from build123d import *

# Parameters (mm, degrees)
SKETCH1_W            = 21.082
SKETCH1_H            = 10.16
BOSS_EXTRUDE1_DEPTH  = 1.651
CUT_EXTRUDE1_DEPTH   = 22.082
MIRROR2_COPY_1_DEPTH = 22.082
CUT_EXTRUDE2_DEPTH   = 11.16
MIRROR4_COPY_1_DEPTH = 11.16
SKETCH4_R            = 0.5
CUT_EXTRUDE3_DEPTH   = 0.1


with BuildPart() as part:
    # Sketch1 → Boss-Extrude1 (new body, symmetric)
    with BuildSketch(Plane(origin=(0, 0, 0), x_dir=(1, 0, 0), z_dir=(0, 1, 0))):
        Rectangle(SKETCH1_W, SKETCH1_H)
    extrude(amount=BOSS_EXTRUDE1_DEPTH, both=True)

    # Sketch2 → Cut-Extrude1 (cut, through all)
    with BuildSketch(Plane(origin=(10.541, 0, 0), x_dir=(0, 0, -1), z_dir=(1, 0, 0))):
        Polygon((-5.08, 1.651), (-4.88, 1.651), (-5.08, 0.1905), align=None)
    cut_extrude1 = extrude(amount=-CUT_EXTRUDE1_DEPTH, mode=Mode.SUBTRACT)

    # Mirror1: Cut-Extrude1 across plane
    add(cut_extrude1.mirror(Plane.XY), mode=Mode.SUBTRACT)

    # Mirror2: Cut-Extrude1 across plane
    add(cut_extrude1.mirror(Plane.ZX), mode=Mode.SUBTRACT)

    # Mirror2 copy 1 sketch → Mirror2 copy 1 (cut, through all)
    with BuildSketch(Plane(origin=(10.541, 0, 0), x_dir=(0, 0, 1), z_dir=(1, 0, 0))):
        Polygon((-5.08, 1.651), (-4.88, 1.651), (-5.08, 0.1905), align=None)
    extrude(amount=-MIRROR2_COPY_1_DEPTH, mode=Mode.SUBTRACT)

    # Sketch3 → Cut-Extrude2 (cut, through all)
    with BuildSketch(Plane.XY.offset(5.08)):
        Polygon((10.541, 0.1905), (10.541, 1.651), (10.341, 1.651), align=None)
    cut_extrude2 = extrude(amount=-CUT_EXTRUDE2_DEPTH, mode=Mode.SUBTRACT)

    # Mirror3: Cut-Extrude2 across plane
    add(cut_extrude2.mirror(Plane.ZX), mode=Mode.SUBTRACT)

    # Mirror4: Cut-Extrude2 across plane
    add(cut_extrude2.mirror(Plane(origin=(0, 0, 0), x_dir=(0, 0, 1), z_dir=(1, 0, 0))), mode=Mode.SUBTRACT)

    # Mirror4 copy 1 sketch → Mirror4 copy 1 (cut, through all)
    with BuildSketch(Plane(origin=(0, 0, 5.08), x_dir=(-1, 0, 0), z_dir=(0, 0, 1))):
        Polygon((10.541, 0.1905), (10.541, 1.651), (10.341, 1.651), align=None)
    extrude(amount=-MIRROR4_COPY_1_DEPTH, mode=Mode.SUBTRACT)

    # Sketch4 → Cut-Extrude3 (cut)
    with BuildSketch(Plane(origin=(0, 1.651, 0), x_dir=(1, 0, 0), z_dir=(0, 1, 0))):
        with Locations((-9.341, -3.88)):
            Circle(SKETCH4_R)
    extrude(amount=-CUT_EXTRUDE3_DEPTH, mode=Mode.SUBTRACT)


solid = part.part
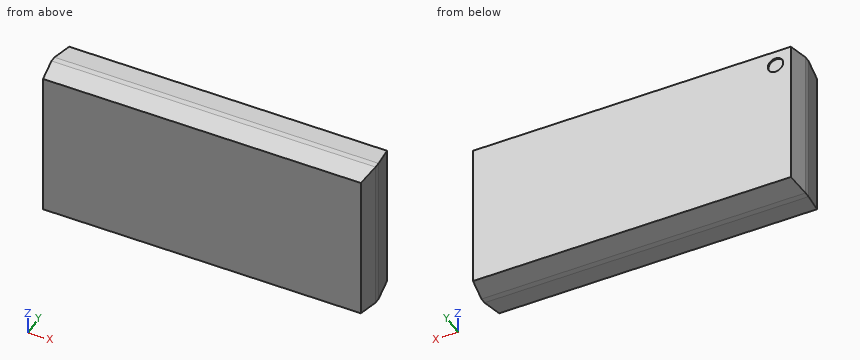
Model file for the job. Use its own axes, mm. Round coordinates to 2 decimals unless told otherwise and drop trailing zeros. Loops run counter-clockwise (first coordinate to the right, second up) from the corner with the lowest first, then second, coordinate; pieces in that order, holes last. Notation, with made-up numbers: M 62.5,46 L 116.5,46 A24 ccw 116.5,84 Z; hole C -23,-38 d5. An arc over 180 degrees is marked long. One line per question, with ' | ' between items.
1) Flat gauge pins, fed straight in: pin 1 (1 mm diameter, centred on y = 1, z = 2, fed in from -X); pin 2 (1.5 mm diameter, centred on x = 7.5, y = 1, fed in from +Z); pin 3 (1 mm diameter, centred on x = -3.5, y = -1, fed in from +Z). Where does each tip first touch, or does it go through?
Solved:
pin 1: stops at x = -10.5 | pin 2: stops at z = 5.07 | pin 3: stops at z = 5.04
2) Band-saw the part on B-B (y = -0.75). Give the cut face in (x, z).
Solved:
outline: M -10.46,-5 L 10.46,-5 L 10.46,5 L -10.46,5 Z
3) Drill centre lines: line 1 along X through (y, z) = (1.6, 3.88); line 2 along Z through (x, y) = (-2, -0.55); line 3 along X through (y, z) = (-0.85, -4.25). Where is each one in solid material? Low to high.
Solved:
line 1: x = -10.35 to -9.84, -8.84 to 10.35 | line 2: z = -5.03 to 5.03 | line 3: x = -10.45 to 10.45
4) Band-saw the part on A-A (x = -4.5). Give the cut face in (y, z), then the cut area to 3 significant figures.
Solved:
outline: M -1.65,-4.88 L -0.19,-5.08 L 0.19,-5.08 L 1.65,-4.88 L 1.65,4.88 L 0.19,5.08 L -0.19,5.08 L -1.65,4.88 Z | area: 33.0 mm²
